Read the model definition and answer for the solid it produces. Units are mm, in the model's axes. Give positions to 0.01 mm unless a question says otherwise; leave off trailing zeros. Order: outer loops, then holes, each group sorted by start corner. A loop starts at its lowest first (then second) coordinate and runs counter-clockwise, first axis right, second up.
Autodesk Inventor part; units mm, degrees
ref_plane "YZ Plane" through (0, 0, 0) normal (1, 0, 0) x (0, 1, 0)
ref_plane "XZ Plane" through (0, 0, 0) normal (0, 1, 0) x (-1, 0, 0)
ref_plane "XY Plane" through (0, 0, 0) normal (0, 0, 1) x (1, 0, 0)
sketch "Sketch1" plane through (0, 0, 0) normal (0, 1, 0) x (-1, 0, 0)
  circle A0 centre (0, 0) radius 50
  circle A1 centre (0, 0) radius 46.5
  circle A2 centre (0, 43.3342) radius 2.375
  line L0 (17.4744, 40) -> (-15.3474, 40)
  line L1 (4, 40) -> (4, 46.3276)
  line L2 (-4, 40) -> (-4, 46.3276)
  line L3 (0, 50) -> (0, 0)
  dimension "d0" = 100
  dimension "d1" = 93
  dimension "d2" = 4.75
  dimension "d6" = 40
  dimension "d8" = 4
  dimension "d10" = 4
  dimension "d11" = 4
  dimension "d12" = 0
extrude "Extrusion1" add sketch "Sketch1" along normal blind 5.5 contours A1 L1 L0 L3 A2 | L3 A2 L0 L2 A1
properties part number "100MagnetHolder_3DPrint"
1) Consider L1, parallel to Z at x = 0, y = 2.25; L2, parallel to X at y = 0.7, z = 44.75; L3, parallel to X at y = 1.2, z = 44.5. Determine where each line is inside the solid, lowest interval first.
Final values:
L1: z = 40 to 40.96, 45.71 to 46.5
L2: x = -4 to -1.91, 1.91 to 4
L3: x = -4 to -2.07, 2.07 to 4
2) The part is cut by section B-B on y = 2.4. Determine the outline of the cut face in (x, z) (3 decimals), and give its area (3 significant figures).
Final values:
outline: (-4, 40) - (4, 40) - (4, 46.328) arc R46.5 ccw to (-4, 46.328) - close; hole circle Ø4.75 at (0, 43.334)
area: 33.8 mm2
3) Given pin 1 (1.5 mm diameter, centred on x = 2, z = 42.5, fed in from +Y), flat-ended and moving along its own axis, determine where the tip first touches the part or whether it passes through.
Final values:
pin 1: stops at y = 5.5
4) The part is cut by section A-A on x = 2.25. Determine the outline of the cut face in (y, z).
Final values:
outline: (0, 40) - (5.5, 40) - (5.5, 42.57) - (0, 42.57) - close; (0, 44.09) - (5.5, 44.09) - (5.5, 46.45) - (0, 46.45) - close
